Check sheet for the modelled part. Datum: model origin and axes. Units: mm. Coordinates: 2 decimals unless noted, no trailing zeros. Write each question's results on one line, items separated by ' | '.
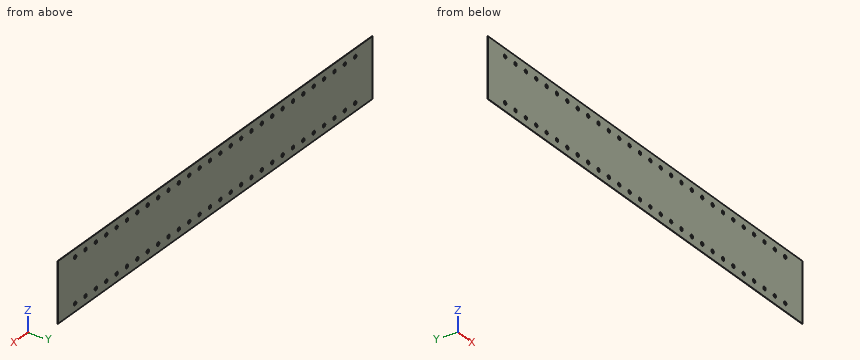
Autodesk Inventor part; units mm, degrees
ref_plane "YZ Plane" through (0, 0, 0) normal (1, 0, 0) x (0, 1, 0)
ref_plane "XZ Plane" through (0, 0, 0) normal (0, 1, 0) x (-1, 0, 0)
ref_plane "XY Plane" through (0, 0, 0) normal (0, 0, 1) x (1, 0, 0)
sketch "Skin Scheme" plane through (0, 0, 0) normal (0, 1, 0) x (-1, 0, 0)
  line L0 (702.5, -84.5) -> (-702.5, -84.5)
  line L1 (-702.5, -84.5) -> (-702.5, 84.5)
  line L2 (-702.5, 84.5) -> (702.5, 84.5)
  line L3 (702.5, 84.5) -> (702.5, -84.5)
  circle A0 centre (580.5, -62.5) radius 5
  circle A1 centre (537.5, -62.5) radius 5
  circle A2 centre (494.5, -62.5) radius 5
  circle A3 centre (451.5, -62.5) radius 5
  circle A4 centre (408.5, -62.5) radius 5
  circle A5 centre (365.5, -62.5) radius 5
  circle A6 centre (322.5, -62.5) radius 5
  circle A7 centre (279.5, -62.5) radius 5
  circle A8 centre (236.5, -62.5) radius 5
  circle A9 centre (193.5, -62.5) radius 5
  circle A10 centre (150.5, -62.5) radius 5
  circle A11 centre (107.5, -62.5) radius 5
  circle A12 centre (64.5, -62.5) radius 5
  circle A13 centre (21.5, -62.5) radius 5
  circle A14 centre (-21.5, -62.5) radius 5
  circle A15 centre (-64.5, -62.5) radius 5
  circle A16 centre (-107.5, -62.5) radius 5
  circle A17 centre (-150.5, -62.5) radius 5
  circle A18 centre (580.5, 62.5) radius 5
  circle A19 centre (537.5, 62.5) radius 5
  circle A20 centre (494.5, 62.5) radius 5
  circle A21 centre (451.5, 62.5) radius 5
  circle A22 centre (408.5, 62.5) radius 5
  circle A23 centre (365.5, 62.5) radius 5
  circle A24 centre (322.5, 62.5) radius 5
  circle A25 centre (279.5, 62.5) radius 5
  circle A26 centre (236.5, 62.5) radius 5
  circle A27 centre (193.5, 62.5) radius 5
  circle A28 centre (150.5, 62.5) radius 5
  circle A29 centre (107.5, 62.5) radius 5
  circle A30 centre (64.5, 62.5) radius 5
  circle A31 centre (21.5, 62.5) radius 5
  circle A32 centre (-21.5, 62.5) radius 5
  circle A33 centre (-64.5, 62.5) radius 5
  circle A34 centre (-107.5, 62.5) radius 5
  circle A35 centre (-150.5, 62.5) radius 5
  circle A36 centre (-193.5, -62.5) radius 5
  circle A37 centre (-193.5, 62.5) radius 5
  circle A38 centre (-236.5, -62.5) radius 5
  circle A39 centre (-236.5, 62.5) radius 5
  circle A40 centre (-279.5, -62.5) radius 5
  circle A41 centre (-279.5, 62.5) radius 5
  circle A42 centre (-322.5, -62.5) radius 5
  circle A43 centre (-322.5, 62.5) radius 5
  circle A44 centre (-365.5, -62.5) radius 5
  circle A45 centre (-365.5, 62.5) radius 5
  circle A46 centre (-408.5, -62.5) radius 5
  circle A47 centre (-408.5, 62.5) radius 5
  circle A48 centre (-451.5, -62.5) radius 5
  circle A49 centre (-451.5, 62.5) radius 5
  circle A50 centre (-494.5, -62.5) radius 5
  circle A51 centre (-494.5, 62.5) radius 5
  circle A52 centre (-537.5, -62.5) radius 5
  circle A53 centre (-537.5, 62.5) radius 5
  circle A54 centre (-580.5, -62.5) radius 5
  circle A55 centre (-580.5, 62.5) radius 5
  point P0 (0, 0)
  dimension "d0" = 1405
  dimension "d1" = 702.5
  dimension "d2" = 169
  dimension "d3" = 84.5
  dimension "d4" = 10
  dimension "d5" = 122
  dimension "d6" = 22
  dimension "d9" = 43
  dimension "d12" = 125
extrude "Skin Body" add sketch "Skin Scheme" along normal blind 1
sketch "End Cut Outline" plane through (0, 1, 0) normal (0, 1, 0) x (1, 0, 0)
  line L0 (-652.5, 94.5) -> (-712.5, 94.5)
  line L1 (-712.5, 94.5) -> (-712.5, -94.5)
  line L2 (-712.5, -94.5) -> (-652.5, -94.5)
  line L3 (-652.5, -94.5) -> (-652.5, 94.5)
  line L4 (702.5, 84.5) -> (-702.5, 84.5)
  line L5 (-702.5, -84.5) -> (702.5, -84.5)
  line L6 (-702.5, 84.5) -> (-702.5, -84.5)
  point P0 (0, 0)
  dimension "d19" = 10
  dimension "d20" = 10
  dimension "d21" = 10
  dimension "d22" = 50
extrude "End Cut" cut sketch "End Cut Outline" along normal through all both and the other way through all
mirror "End Cut Mirror" about plane through (0, 0, 0) normal (1, 0, 0) of "End Cut"
properties part number "Skin NPS 12 Internal" material "Rubber, Silicone"
1. Material ranges on L1, parallel to Z at x = 21.5, y = 0.4; L2, parallel to Z at x = -19.5, y = 0.1, recorded low to high. Write a range as [from, to].
Values follow:
L1: z = [-84.5, -67.5], [-57.5, 57.5], [67.5, 84.5] | L2: z = [-84.5, -67.08], [-57.92, 57.92], [67.08, 84.5]
2. Sectioned sample at A-A (y = 0.7). Give the number of separate pieces and of enclosed holes in the cut face, then the cut area to 3 significant figures.
Values follow:
separate pieces: 1 | enclosed holes: 56 | area: 216,000 mm^2
3. Go/stop test with flat-tipped pins: pin 1 (8 mm diameter, centred on x = 229.5, z = 12, fed in from -Y); pin 2 (9 mm diameter, centred on x = 150.5, z = -62.5, fed in from +Y). Record where each tip stops, or that it passes through.
Values follow:
pin 1: stops at y = 0 | pin 2: passes through
